Geometry: final body of the model. Coordinates: model frame, mm. A direction names the side the tool comes from. Coordinates: 2 decimals unless noted, no trailing zeros. Order: outer loops, then holes, each group sorted by start corner. A loop starts at its lowest first (then second) coordinate and runs counter-clockwise, first axis right, second up. Notation, with made-up numbers: M -20,16 L -14,16 A11 cw -14,30 Z; hole C 40,-1 d8. An arc over 180 degrees is marked long. Write item = value, one per line. Start each with the question number.
```python
from build123d import *

# Parameters (mm, degrees)
EXTRUDE_1_DEPTH     = 12.5
SKETCH_2_W          = 32
SKETCH_2_H          = 32
EXTRUDE_2_DEPTH     = 5
CHAMFER_1_SIZE      = 1
CHAMFER_2_SIZE      = 1
SKETCH_3_R          = 2.75
CUT_EXTRUDE_1_DEPTH = 46.194717612
CHAMFER_3_SIZE      = 1
SKETCH_4_R          = 6
CUT_EXTRUDE_2_DEPTH = 49.141068746
SKETCH_5_R          = 11
CUT_EXTRUDE_3_DEPTH = 3


with BuildPart() as part:
    # Sketch 1 → Extrude 1 (new, symmetric)
    with BuildSketch(Plane.XY):
        Polygon((-30, 16.25), (-30, -16.25), (30, -16.25), (30, 16.25), (17, 16.25), (17, 22.75), (-17, 22.75), (-17, 16.25), align=None)
    extrude(amount=EXTRUDE_1_DEPTH, both=True)

    # Sketch 2 → Extrude 2 (add)
    with BuildSketch(Plane.XY.offset(12.5)):
        with Locations((0, 5.75)):
            Rectangle(SKETCH_2_W, SKETCH_2_H)
    extrude(amount=EXTRUDE_2_DEPTH)

    # Chamfer 1
    chamfer_1_edges = [part.edges().sort_by_distance(p)[0] for p in [
        (-16, 21.75, 15),
        (-16, -10.25, 15),
        (16, -10.25, 15),
        (16, 21.75, 15),
    ]]
    chamfer(chamfer_1_edges, length=CHAMFER_1_SIZE)

    # Chamfer 2
    chamfer_2_edges = [part.edges().sort_by_distance(p)[0] for p in [
        (30, 16.25, 0),
        (-30, 16.25, 0),
    ]]
    chamfer(chamfer_2_edges, length=CHAMFER_2_SIZE)

    # Sketch 3 → Cut-Extrude 1 (cut, through all)
    with BuildSketch(Plane.XY.offset(12.5)):
        with Locations((-23, 8.75)):
            Circle(SKETCH_3_R)
        with Locations((-23, -9.25)):
            Circle(SKETCH_3_R)
    cut_extrude_1 = extrude(amount=-CUT_EXTRUDE_1_DEPTH, mode=Mode.SUBTRACT)

    # Mirror 1: Cut-Extrude 1 across plane
    add(cut_extrude_1.mirror(Plane(origin=(0, 0, 0), x_dir=(0, 0, 1), z_dir=(1, 0, 0))), mode=Mode.SUBTRACT)

    # Chamfer 3
    chamfer_3_edges = [part.edges().sort_by_distance(p)[0] for p in [
        (-17, 22.75, 0),
        (17, 22.75, 0),
    ]]
    chamfer(chamfer_3_edges, length=CHAMFER_3_SIZE)

    # Sketch 4 → Cut-Extrude 2 (cut, through all)
    with BuildSketch(Plane.XY.offset(17.5)):
        with Locations((0, 4.75)):
            Circle(SKETCH_4_R)
    extrude(amount=-CUT_EXTRUDE_2_DEPTH, mode=Mode.SUBTRACT)

    # Sketch 5 → Cut-Extrude 3 (cut)
    with BuildSketch(Plane.XY.offset(17.5)):
        with Locations((0, 4.75)):
            Circle(SKETCH_5_R)
    extrude(amount=-CUT_EXTRUDE_3_DEPTH, mode=Mode.SUBTRACT)


solid = part.part
```
Item 1: Section query A-A on y = 4.75. Output: boundary loops of the cut face in (x, z), and give its area (3 significant figures).
Item 2: Reachability of faces 1 (the flat face through (-16, 6, 15)), 2 (the flat face through (0, 21.75, 15)), 3 (the flat face through (16, 6, 15)), 4 (the flat face through (-17, 19, 0)), 5 (the flat face through (5, 0, 14.5)) from +Z, -Z, +X, -X, +Y, -Y: full face, straight path, thin tool, end or side. Return the list, or none.
Item 3: Section query C-C on x = 23. Output: boundary loops of the cut face in (y, z).
Item 4: Material intervals for probe 1 along Y at (x, z) = (23, 0); probe 2 along X at (y, z) = (11, 3.25); probe 3 along Z at (x, y) = (-4, -13.5), sorted ascending. Write a range as [from, to].
Item 5: First-contact query: pin 1 (6 mm diameter, centred on y = 18.5, z = -3.5, fed in from -X); pin 2 (9.5 mm diameter, centred on x = 21, z = 5.5, fed in from +Y); pin 3 (3 mm diameter, centred on x = -21.5, z = -8, fed in from +Y); pin 4 (1.5 mm diameter, centred on x = -7.5, y = 12.5, fed in from +Z). Flat tips, straight axial feed; report the tip coordinate or a pass-through.
Item 6: Section query D-D on z = 4. Output: boundary loops of the cut face in (x, y), and give its area (3 significant figures).
Item 7: Section query B-B on x = 0. Output: boundary loops of the cut face in (y, z), and give its area (3 significant figures).
Item 8: Draft query along Y for faces 6 (the cylindrical face through (-2.38, -5.99, 16.02)), 7 (the flat face through (0, -16.25, 0)), 8 (the flat face through (0, 22.75, 0)). Return one class per face: pulls with the +Y half, pulls with the -Y half, needs draft (parallel to the pull), parting line crosses it, or undercut.
Ans:
q1.outline = M -30,-12.5 L -6,-12.5 L -6,14.5 L -11,14.5 L -11,17.5 L -16,17.5 L -16,12.5 L -30,12.5 Z; M 6,-12.5 L 30,-12.5 L 30,12.5 L 16,12.5 L 16,17.5 L 11,17.5 L 11,14.5 L 6,14.5 Z
q1.area = 1,270 mm^2
q2.face_1 = +Z, -X, +Y, -Y
q2.face_2 = +Z, +X, -X, +Y
q2.face_3 = +Z, +X, +Y, -Y
q2.face_4 = +Z, -Z, -X, +Y
q2.face_5 = +Z
q3.outline = M -16.25,-12.5 L -12,-12.5 L -12,12.5 L -16.25,12.5 Z; M -6.5,-12.5 L 6,-12.5 L 6,12.5 L -6.5,12.5 Z; M 11.5,-12.5 L 16.25,-12.5 L 16.25,12.5 L 11.5,12.5 Z
q4.probe_1 = [-16.25, -12], [-6.5, 6], [11.5, 16.25]
q4.probe_2 = [-30, -24.58], [-21.42, 21.42], [24.58, 30]
q4.probe_3 = [-12.5, 12.5]
q5.pin_1 = -29.75
q5.pin_2 = 22.5
q5.pin_3 = 16.25
q5.pin_4 = 17.5
q6.outline = M -30,-16.25 L 30,-16.25 L 30,15.25 L 29,16.25 L 17,16.25 L 17,21.75 L 16,22.75 L -16,22.75 L -17,21.75 L -17,16.25 L -29,16.25 L -30,15.25 Z; hole C -23,-9.25 d5.5; hole C -23,8.75 d5.5; hole C 0,4.75 d12; hole C 23,-9.25 d5.5; hole C 23,8.75 d5.5
q6.area = 1,960 mm^2
q7.outline = M -16.25,-12.5 L -1.25,-12.5 L -1.25,14.5 L -6.25,14.5 L -6.25,17.5 L -10.25,17.5 L -10.25,12.5 L -16.25,12.5 Z; M 10.75,-12.5 L 22.75,-12.5 L 22.75,12.5 L 21.75,12.5 L 21.75,17.5 L 15.75,17.5 L 15.75,14.5 L 10.75,14.5 Z
q7.area = 745 mm^2
q8.face_6 = undercut
q8.face_7 = pulls with the -Y half
q8.face_8 = pulls with the +Y half
